Could you check a few things on this drawing? It's one solid part, dimensions in mm from its lowest x, y, z. Round coordinates to 2 decimals unless told otherwise and drop trailing zeros. Write each loop counter-clockwise with the first axis right and the second up, starting at its lowest first coordinate (ties: lowest second). Pieces come first, ordered by that corner, then holes. Notation, with made-up numbers: (-12.5, 29) -> (9.5, 29) arc R25 ccw to (9.5, 45) -> close; hole circle Ø1 at (49.25, 56). An arc over 180 degrees is marked (long way). Answer in a Markdown table with one row per item. Add a question column.
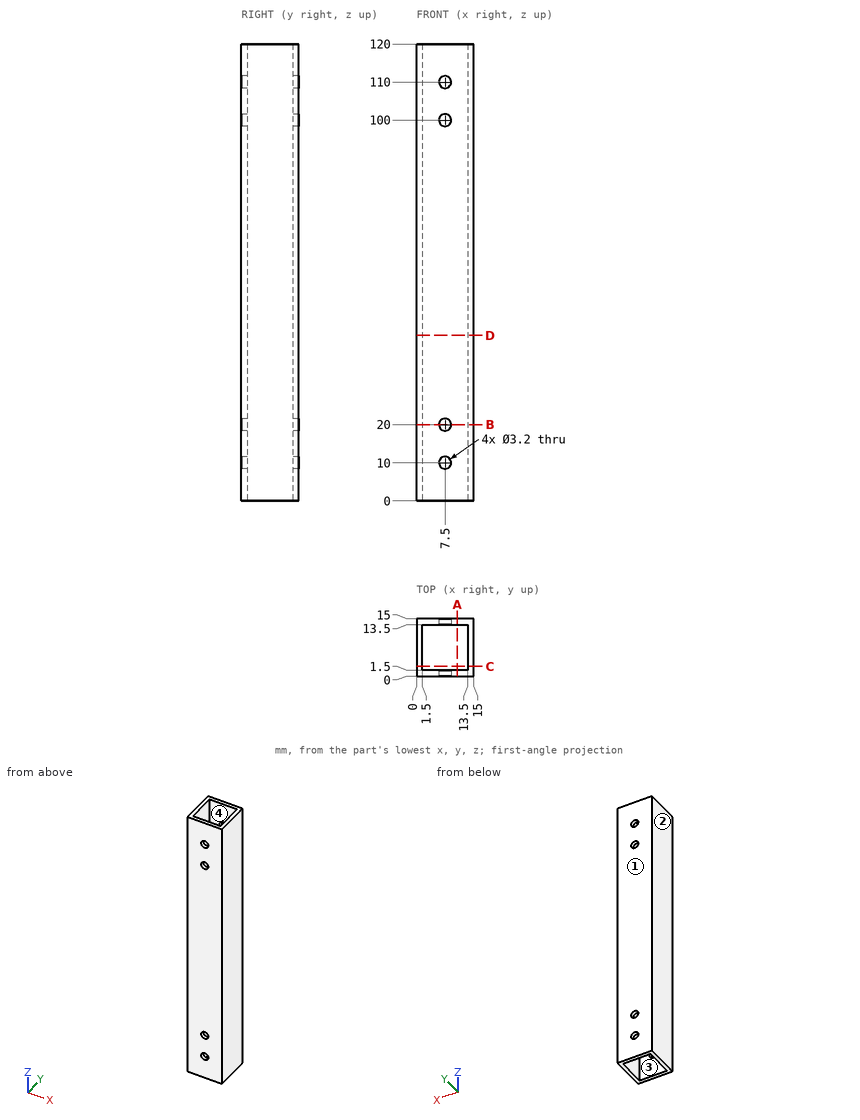
Item 1: If we mould it in two halves opening along Y, with no side actions, what happens to the marked faces 1, 2, 3 and 4? For each: pulls with the +Y half, pulls with the -Y half, needs draft (parallel to the pull), parting line crosses it, or undercut.
Item 2: If we section it at B-B on z = 20: Please give me the cut outline in (x, y), then the cut area to 3 significant figures.
Item 3: If we section it at A-A on x = 10.75: Please give me the cut outline in (y, z).
Item 4: If we section it at D-D on z = 43.5: Please give me the cut outline in (x, y), then the cut area to 3 significant figures.
Item 5: I need wall thicknesses on line 1 along Z through (x, y) = (7.5, 14.2); line 2 along Y through (x, z) = (2.75, 42). Which ranges of each line are inside material? Lowest first, please. Write a range as from..to.
Results list:
| question | item | result |
|---|---|---|
| 1 | face 1 | pulls with the +Y half |
| 1 | face 2 | needs draft |
| 1 | face 3 | undercut |
| 1 | face 4 | undercut |
| 2 | outline | (0, 0) -> (5.9, 0) -> (5.9, 1.5) -> (1.5, 1.5) -> (1.5, 13.5) -> (5.9, 13.5) -> (5.9, 15) -> (0, 15) -> close; (9.1, 0) -> (15, 0) -> (15, 15) -> (9.1, 15) -> (9.1, 13.5) -> (13.5, 13.5) -> (13.5, 1.5) -> (9.1, 1.5) -> close |
| 2 | area | 71.4 mm² |
| 3 | outline | (0, 0) -> (1.5, 0) -> (1.5, 120) -> (0, 120) -> close; (13.5, 0) -> (15, 0) -> (15, 120) -> (13.5, 120) -> close |
| 4 | outline | (0, 0) -> (15, 0) -> (15, 15) -> (0, 15) -> close; hole (1.5, 1.5) -> (13.5, 1.5) -> (13.5, 13.5) -> (1.5, 13.5) -> close |
| 4 | area | 81.0 mm² |
| 5 | line 1 | 0..8.4, 11.6..18.4, 21.6..98.4, 101.6..108.4, 111.6..120 |
| 5 | line 2 | 0..1.5, 13.5..15 |
